Verification items for the finished model (mm, model axes). A direction names the side the tool comes from. Round coordinates to 2 decimals unless told otherwise and drop trailing zeros. Loops run counter-clockwise (first coordinate to the right, second up) from the corner with the lowest first, then second, coordinate; pieces in that order, holes last. Notation, with made-up numbers: M -31,20 L -12,20 A36 cw -12,59 Z; hole C -34,59.5 d2. An arc over 180 degrees is marked long. Answer as CSV lines item,"result".
Autodesk Inventor part; units mm, degrees
ref_plane "YZ Plane" through (0, 0, 0) normal (1, 0, 0) x (0, 1, 0)
ref_plane "XZ Plane" through (0, 0, 0) normal (0, 1, 0) x (-1, 0, 0)
ref_plane "XY Plane" through (0, 0, 0) normal (0, 0, 1) x (1, 0, 0)
sketch "Эскиз1" plane through (0, 0, 0) normal (0, 0, 1) x (1, 0, 0)
  line L0 (17.5, 5) -> (-17.5, 5) construction
  line L1 (-17.5, 5) -> (-17.5, -5) construction
  line L2 (-17.5, -5) -> (17.5, -5) construction
  line L3 (17.5, -5) -> (17.5, 5) construction
  line L4 (17.5, 5) -> (-17.5, -5) construction
  line L5 (-17.5, 5) -> (17.5, -5) construction
  line L6 (12.8471, 5) -> (-11.1661, 5) construction
  circle A0 centre (0, 64.187) radius 35
  circle A1 centre (0, 64.187) radius 20
  line L7 (0, 64.187) -> (0, 0) construction
  circle A2 centre (0, 88.737) radius 4.55
  line L8 (-7.5, 5) -> (-7.5, 30)
  line L9 (7.5, 30) -> (7.5, 5)
  line L10 (-2, 49.2906) -> (2, 49.2906) construction
  line L11 (-7.5, 5) -> (7.5, 5)
  line L12 (-2, 85.687) -> (2, 85.687)
  line L13 (2, 85.687) -> (2, 82.687)
  line L14 (2, 82.687) -> (-2, 82.687)
  line L15 (-2, 82.687) -> (-2, 85.687)
  line L16 (-2, 85.687) -> (2, 82.687) construction
  line L17 (2, 85.687) -> (-2, 82.687) construction
  line L18 (-17.6195, 51.7049) -> (-19.6195, 55.169)
  circle A3 centre (-21.2609, 51.912) radius 4.55
  line L19 (-17.0215, 56.669) -> (-15.0215, 53.2049)
  line L20 (-19.6195, 55.169) -> (-17.0215, 56.669)
  line L21 (-15.0215, 53.2049) -> (-17.6195, 51.7049)
  line L22 (19.6195, 55.169) -> (17.6195, 51.7049)
  circle A4 centre (21.2609, 51.912) radius 4.55
  line L23 (15.0215, 53.2049) -> (17.0215, 56.669)
  line L24 (17.6195, 51.7049) -> (15.0215, 53.2049)
  line L25 (17.0215, 56.669) -> (19.6195, 55.169)
  point P0 (0, 89.2906)
  point P1 (0, 84.187)
  point P2 (-17.3205, 54.187)
  point P3 (17.3205, 54.187)
  point P4 (18.2337, 55.9692)
  point P5 (18.7216, 55.6875)
  point P6 (16.7216, 52.2234)
  point P7 (16.2337, 52.5051)
  point P8 (-16.2337, 52.5051)
  point P9 (-16.7216, 52.2234)
  point P10 (-18.7216, 55.6875)
  point P11 (-18.2337, 55.9692)
  point P12 (-2, 84.0867)
  point P13 (-2, 84.6501)
  point P14 (2, 84.6501)
  point P15 (2, 84.0867)
  dimension "d3" = 40
  dimension "d4" = 9.1
  dimension "d0" = 70
  dimension "d9" = 35
  dimension "d10" = 25
  dimension "d11" = 10
  dimension "d12" = 15
  dimension "d14" = 7.5
  dimension "d30" = 4
  dimension "d31" = 3
  dimension "d34" = 360
extrude "Выдавливание1" add sketch "Эскиз1" along normal blind 3
fillet "Сопряжение1" radius 2 14 edges at (-7.5, 30, 1.5) (7.5, 30, 1.5) (-18.2337, 55.9692, 1.5) (-18.7216, 55.6875, 1.5) (-16.2337, 52.5051, 1.5) (-16.7216, 52.2234, 1.5) (-2, 84.0867, 1.5) (-2, 84.6501, 1.5) (2, 84.0867, 1.5) (2, 84.6501, 1.5) (18.7216, 55.6875, 1.5) (18.2337, 55.9692, 1.5) (16.7216, 52.2234, 1.5) (16.2337, 52.5051, 1.5)
sketch "Эскиз2" plane through (0, 0, 3) normal (0, 0, 1) x (1, 0, 0)
  circle A0 centre (0, 25) radius 1.5
  circle A1 centre (0, 10) radius 2.5
  line L0 (0, 0) -> (0, 43.9437)
  line L1 (0, 10) -> (0, 5)
  line L2 (-7.5, 5) -> (7.5, 5)
  dimension "d24" = 15
  dimension "d25" = 5
  dimension "d26" = 5
  dimension "d27" = 3
extrude "Выдавливание2" cut sketch "Эскиз2" against normal blind 4
properties part number "Деталь1_мозговорот"
1) Go/stop test with flat-tipped pins: pin 1 (1.5 mm diameter, centred on x = -12.5, z = 0.5, fed in from -Y); pin 2 (1 mm diameter, centred on x = 8.5, z = 1.5, fed in from -Y); pin 3 (1.5 mm diameter, centred on x = -24, z = 2, fed in from +Y). Record where each tip stops, or that it passes through.
Here are the results:
pin 1,"stops at y = 31.22"
pin 2,"stops at y = 29.75"
pin 3,"stops at y = 90.35"
2) Set-up check for faces 1 (the flat face through (0, 42, 0)), 2 (the cylindrical face through (17.209, 74.377, 1.479)): record each of +Z, -Z, +X, -X, +Y, -Y from which the full face is reachable in a straight line by a thin tool's end or side.
Here are the results:
face 1,"-Z, +X, -X, +Y, -Y"
face 2,"+Z, -Z"
3) Section check D-D (y = 10). Record the cut outline in (x, z).
Here are the results:
outline,"M -7.5,0 L -2.5,0 L -2.5,3 L -7.5,3 Z; M 2.5,0 L 7.5,0 L 7.5,3 L 2.5,3 Z"
4) Material ranges on probe 1 along Y at (x, z) = (0, 0.75); probe 2 along X at (y, z) = (10, 1.2); probe 3 along X at (y, z) = (25, 2), recorded low to high.
Here are the results:
probe 1,"y = 5 to 7.5, 12.5 to 23.5, 26.5 to 44.19, 93.29 to 99.19"
probe 2,"x = -7.5 to -2.5, 2.5 to 7.5"
probe 3,"x = -7.5 to -1.5, 1.5 to 7.5"
5) Section check A-A (y = 25). Record the cut outline in (x, z), plus the area to 3 significant figures.
Here are the results:
outline,"M -7.5,0 L -1.5,0 L -1.5,3 L -7.5,3 Z; M 1.5,0 L 7.5,0 L 7.5,3 L 1.5,3 Z"
area,"36.0 mm^2"
6) Section check B-B (x = 0). Record the cut outline in (y, z), plus the area to 3 significant figures.
Here are the results:
outline,"M 5,0 L 7.5,0 L 7.5,3 L 5,3 Z; M 12.5,0 L 23.5,0 L 23.5,3 L 12.5,3 Z; M 26.5,0 L 44.19,0 L 44.19,3 L 26.5,3 Z; M 93.29,0 L 99.19,0 L 99.19,3 L 93.29,3 Z"
area,"111 mm^2"
7) Draft check along Y on faces 3 (the flat face through (-7.5, 17, 1)), 4 (the cylindrical face through (-7.926, 29.661, 1.479)), 5 (the cylindrical face through (-15.867, 50.633, 1.479)). Enter one of: +Y half, -Y half, draft (parallel to the pull), parting line (faces both ways), or undercut.
Here are the results:
face 3,"draft"
face 4,"-Y half"
face 5,"undercut"
8) Section check C-C (z = 0.65). Record the cut outline in (x, y).
Here are the results:
outline,"M -8.99,30.36 A2 cw -7.5,28.43 L -7.5,5 L 7.5,5 L 7.5,28.43 A2 cw 8.99,30.36 A35 ccw long Z; hole M -21.25,56.46 A4.55 ccw long -17.31,49.65 A2 cw -14.16,50.07 A20 ccw 14.16,50.07 A2 cw 17.31,49.65 A4.55 ccw long 21.25,56.46 A2 cw 19.31,58.98 A20 ccw 5.15,83.51 A2 cw 3.93,86.45 A4.55 ccw long -3.93,86.45 A2 cw -5.15,83.51 A20 ccw -19.31,58.98 A2 cw Z; hole C 0,10 d5; hole C 0,25 d3"
